Verification items for the finished model (mm, model axes). A direction names the side the tool comes from. Coordinates: 2 decimals unless noted, no trailing zeros. Loops run counter-clockwise (first coordinate to the right, second up) from the corner with the lowest first, then second, coordinate; pieces in that order, holes last. Notation, with made-up numbers: (-31.5, 41) - (-10.5, 41) arc R15 ccw to (-10.5, 52) - close; hole circle Ø5 at (20.25, 62). An arc over 180 degrees is marked (long way). Answer as CSV lines item,"result". Start each with the question number.
1. Cross-section at C-C (z = 45.5). Enter the section's corners in (x, y), plus the area to 3 significant figures.
2. Cross-section at A-A (z = 0). Enter the section's corners in (x, y), plus the area to 3 significant figures.
3. Set-up check for faces 5 (the flat face through (-63.292, -153, 29)), 6 (the flat face through (-54.96, -150.6, 51.33)), 7 (the flat face through (-63.292, -153, -30)), 8 (the flat face through (-65, -150, 0)): record each of +Z, -Z, +X, -X, +Y, -Y from which the full face is reachable in a straight line by a thin tool's end or side.
4. Gauge pin test, flat ends, axial feed: P1, Ø4, axis at x = -101, y = -151, coming from the -Z side; P2, Ø4, axis at x = -56.29, z = 50, coming from the +Y side; P3, Ø1.8, axis at x = -56, z = -9, coming from the -Y side; P4, Ø11, axis at x = -56.29, z = 0, coming from the -Y side. Record the tip position at first contact, or that the pin passes through.
5. Material ranges on line 1 (X direction, y = -149.65, z = 0); line 2 (X direction, y = -153.95, z = 0); line 3 (X direction, y = -150.15, z = 0), recorded low to high. Write a range as [from, to].
6. Release check for a two-part mould opening along Z. For faces 1 (the cylindrical face through (-56.4, -153.1, 57)), 2 (the cylindrical face through (-109.32, -149.81, -0.67)), 3 (the flat face through (-49.292, -153, -29)), 4 (the flat face through (-85, -153, -7)) record: pulls with the +Z half, pulls with the -Z half, needs draft (parallel to the pull), parting line crosses it, or undercut.
7. Cross-section at B-B (x = -72). Enter the section's corners in (y, z).
```python
from build123d import *

# Parameters (mm, degrees)
BASE_OUTLINE_SKETCH_R          = 1.7
BASE_OUTLINE_SKETCH_R_2        = 6.1
BASE_OUTLINE_SKETCH_R_3        = 1.6
BASE_OUTLINE_DEPTH             = 4
INTERFACE_PROFILE_2_SKETCH_R   = 1.7
INTERFACE_PROFILE_2_SKETCH_R_2 = 6.1
INTERFACE_PROFILE_2_SKETCH_R_3 = 1.1
INTERFACE_PROFILE_2_DEPTH      = 2.4
INTERFACE_PROFILE_3_SKETCH_R   = 6.1
INTERFACE_PROFILE_3_SKETCH_R_2 = 3.1
INTERFACE_PROFILE_3_SKETCH_R_3 = 1.1
INTERFACE_PROFILE_3_DEPTH      = 0.6
INTERFACE_PROFILE_4_SKETCH_R   = 6.1
INTERFACE_PROFILE_4_SKETCH_R_2 = 3.1
INTERFACE_PROFILE_4_DEPTH      = 1


with BuildPart() as part:
    # Base Outline Sketch → Base Outline (new body)
    with BuildSketch(Plane(origin=(0, -157, 0), x_dir=(1, 0, 0), z_dir=(0, 1, 0))):
        with BuildLine():
            Line((-106.291651246, -7), (-64.77693262, -7))
            ThreePointArc((-64.77693262, -7), (-64.069825839, -7.778174593), (-63.291651246, -8.485281374))
            Line((-63.291651246, -8.485281374), (-63.291651246, -50))
            ThreePointArc((-63.291651246, -50), (-56.291651246, -57), (-49.291651246, -50))
            Line((-49.291651246, -50), (-49.291651246, -8.485281374))
            ThreePointArc((-49.291651246, -8.485281374), (-45.291651246, 0), (-49.291651246, 8.485281374))
            Line((-49.291651246, 8.485281374), (-49.291651246, 50))
            ThreePointArc((-49.291651246, 50), (-56.291651246, 57), (-63.291651246, 50))
            Line((-63.291651246, 50), (-63.291651246, 8.485281374))
            ThreePointArc((-63.291651246, 8.485281374), (-64.069825839, 7.778174593), (-64.77693262, 7))
            Line((-64.77693262, 7), (-106.291651246, 7))
            ThreePointArc((-106.291651246, 7), (-113.291651246, 0), (-106.291651246, -7))
        make_face()
        with Locations(Location((-106.291651246, 0, 0), (0, 0, 270))):
            Circle(BASE_OUTLINE_SKETCH_R, mode=Mode.SUBTRACT)
        with Locations(Location((-56.291651246, 50, 0), (0, 0, 270))):
            Circle(BASE_OUTLINE_SKETCH_R, mode=Mode.SUBTRACT)
        with Locations(Location((-56.291651246, 0, 0), (0, 0, 270))):
            Circle(BASE_OUTLINE_SKETCH_R_2, mode=Mode.SUBTRACT)
        with Locations(Location((-56.291651246, -50, 0), (0, 0, 270))):
            Circle(BASE_OUTLINE_SKETCH_R, mode=Mode.SUBTRACT)
        with Locations(Location((-65.291651246, 0, 0), (0, 0, 270))):
            Circle(BASE_OUTLINE_SKETCH_R_3, mode=Mode.SUBTRACT)
        with Locations(Location((-56.291651246, -9, 0), (0, 0, 270))):
            Circle(BASE_OUTLINE_SKETCH_R_3, mode=Mode.SUBTRACT)
        with Locations(Location((-56.291651246, 9, 0), (0, 0, 270))):
            Circle(BASE_OUTLINE_SKETCH_R_3, mode=Mode.SUBTRACT)
    extrude(amount=BASE_OUTLINE_DEPTH)

    # Interface Profile 2 Sketch → Interface Profile 2 (add)
    with BuildSketch(Plane(origin=(0, -153, 0), x_dir=(1, 0, 0), z_dir=(0, 1, 0))):
        with BuildLine():
            Line((-106.291651246, -7), (-64.77693262, -7))
            ThreePointArc((-64.77693262, -7), (-64.069825839, -7.778174593), (-63.291651246, -8.485281374))
            Line((-63.291651246, -8.485281374), (-63.291651246, -50))
            ThreePointArc((-63.291651246, -50), (-56.291651246, -57), (-49.291651246, -50))
            Line((-49.291651246, -50), (-49.291651246, -8.485281374))
            ThreePointArc((-49.291651246, -8.485281374), (-45.291651246, 0), (-49.291651246, 8.485281374))
            Line((-49.291651246, 8.485281374), (-49.291651246, 50))
            ThreePointArc((-49.291651246, 50), (-56.291651246, 57), (-63.291651246, 50))
            Line((-63.291651246, 50), (-63.291651246, 8.485281374))
            ThreePointArc((-63.291651246, 8.485281374), (-64.069825839, 7.778174593), (-64.77693262, 7))
            Line((-64.77693262, 7), (-106.291651246, 7))
            ThreePointArc((-106.291651246, 7), (-113.291651246, 0), (-106.291651246, -7))
        make_face()
        with Locations(Location((-106.291651246, 0, 0), (0, 0, 270))):
            Circle(INTERFACE_PROFILE_2_SKETCH_R, mode=Mode.SUBTRACT)
        with Locations(Location((-56.291651246, 50, 0), (0, 0, 270))):
            Circle(INTERFACE_PROFILE_2_SKETCH_R, mode=Mode.SUBTRACT)
        with Locations(Location((-56.291651246, 0, 0), (0, 0, 270))):
            Circle(INTERFACE_PROFILE_2_SKETCH_R_2, mode=Mode.SUBTRACT)
        with Locations(Location((-56.291651246, -50, 0), (0, 0, 270))):
            Circle(INTERFACE_PROFILE_2_SKETCH_R, mode=Mode.SUBTRACT)
        with Locations(Location((-65.291651246, 0, 0), (0, 0, 270))):
            Circle(INTERFACE_PROFILE_2_SKETCH_R_3, mode=Mode.SUBTRACT)
        with Locations(Location((-56.291651246, -9, 0), (0, 0, 270))):
            Circle(INTERFACE_PROFILE_2_SKETCH_R_3, mode=Mode.SUBTRACT)
        with Locations(Location((-56.291651246, 9, 0), (0, 0, 270))):
            Circle(INTERFACE_PROFILE_2_SKETCH_R_3, mode=Mode.SUBTRACT)
    extrude(amount=INTERFACE_PROFILE_2_DEPTH)

    # Interface Profile 3 Sketch → Interface Profile 3 (add)
    with BuildSketch(Plane(origin=(0, -150.6, 0), x_dir=(1, 0, 0), z_dir=(0, 1, 0))):
        with BuildLine():
            Line((-106.291651246, -7), (-64.77693262, -7))
            ThreePointArc((-64.77693262, -7), (-64.069825839, -7.778174593), (-63.291651246, -8.485281374))
            Line((-63.291651246, -8.485281374), (-63.291651246, -50))
            ThreePointArc((-63.291651246, -50), (-56.291651246, -57), (-49.291651246, -50))
            Line((-49.291651246, -50), (-49.291651246, -8.485281374))
            ThreePointArc((-49.291651246, -8.485281374), (-45.291651246, 0), (-49.291651246, 8.485281374))
            Line((-49.291651246, 8.485281374), (-49.291651246, 50))
            ThreePointArc((-49.291651246, 50), (-56.291651246, 57), (-63.291651246, 50))
            Line((-63.291651246, 50), (-63.291651246, 8.485281374))
            ThreePointArc((-63.291651246, 8.485281374), (-64.069825839, 7.778174593), (-64.77693262, 7))
            Line((-64.77693262, 7), (-106.291651246, 7))
            ThreePointArc((-106.291651246, 7), (-113.291651246, 0), (-106.291651246, -7))
        make_face()
        with Locations(Location((-56.291651246, 0, 0), (0, 0, 270))):
            Circle(INTERFACE_PROFILE_3_SKETCH_R, mode=Mode.SUBTRACT)
        with Locations(Location((-106.291651246, 0, 0), (0, 0, 270))):
            Circle(INTERFACE_PROFILE_3_SKETCH_R_2, mode=Mode.SUBTRACT)
        with Locations(Location((-56.291651246, 50, 0), (0, 0, 270))):
            Circle(INTERFACE_PROFILE_3_SKETCH_R_2, mode=Mode.SUBTRACT)
        with Locations(Location((-56.291651246, -50, 0), (0, 0, 270))):
            Circle(INTERFACE_PROFILE_3_SKETCH_R_2, mode=Mode.SUBTRACT)
        with Locations(Location((-65.291651246, 0, 0), (0, 0, 270))):
            Circle(INTERFACE_PROFILE_3_SKETCH_R_3, mode=Mode.SUBTRACT)
        with Locations(Location((-56.291651246, -9, 0), (0, 0, 270))):
            Circle(INTERFACE_PROFILE_3_SKETCH_R_3, mode=Mode.SUBTRACT)
        with Locations(Location((-56.291651246, 9, 0), (0, 0, 270))):
            Circle(INTERFACE_PROFILE_3_SKETCH_R_3, mode=Mode.SUBTRACT)
    extrude(amount=INTERFACE_PROFILE_3_DEPTH)

    # Interface Profile 4 Sketch → Interface Profile 4 (add)
    with BuildSketch(Plane(origin=(0, -150, 0), x_dir=(1, 0, 0), z_dir=(0, 1, 0))):
        with BuildLine():
            Line((-106.291651246, -7), (-64.77693262, -7))
            ThreePointArc((-64.77693262, -7), (-64.069825839, -7.778174593), (-63.291651246, -8.485281374))
            Line((-63.291651246, -8.485281374), (-63.291651246, -50))
            ThreePointArc((-63.291651246, -50), (-56.291651246, -57), (-49.291651246, -50))
            Line((-49.291651246, -50), (-49.291651246, -8.485281374))
            ThreePointArc((-49.291651246, -8.485281374), (-45.291651246, 0), (-49.291651246, 8.485281374))
            Line((-49.291651246, 8.485281374), (-49.291651246, 50))
            ThreePointArc((-49.291651246, 50), (-56.291651246, 57), (-63.291651246, 50))
            Line((-63.291651246, 50), (-63.291651246, 8.485281374))
            ThreePointArc((-63.291651246, 8.485281374), (-64.069825839, 7.778174593), (-64.77693262, 7))
            Line((-64.77693262, 7), (-106.291651246, 7))
            ThreePointArc((-106.291651246, 7), (-113.291651246, 0), (-106.291651246, -7))
        make_face()
        with Locations(Location((-56.291651246, 0, 0), (0, 0, 270))):
            Circle(INTERFACE_PROFILE_4_SKETCH_R, mode=Mode.SUBTRACT)
        with Locations(Location((-106.291651246, 0, 0), (0, 0, 270))):
            Circle(INTERFACE_PROFILE_4_SKETCH_R_2, mode=Mode.SUBTRACT)
        with Locations(Location((-56.291651246, 50, 0), (0, 0, 270))):
            Circle(INTERFACE_PROFILE_4_SKETCH_R_2, mode=Mode.SUBTRACT)
        with Locations(Location((-56.291651246, -50, 0), (0, 0, 270))):
            Circle(INTERFACE_PROFILE_4_SKETCH_R_2, mode=Mode.SUBTRACT)
    extrude(amount=INTERFACE_PROFILE_4_DEPTH)


solid = part.part
```
Values follow:
1,outline,"(-63.29, -157) - (-49.29, -157) - (-49.29, -149) - (-63.29, -149) - close"
1,area,"112 mm²"
2,outline,"(-113.29, -157) - (-107.99, -157) - (-107.99, -150.6) - (-109.39, -150.6) - (-109.39, -149) - (-113.29, -149) - close; (-104.59, -157) - (-66.89, -157) - (-66.89, -153) - (-66.39, -153) - (-66.39, -150) - (-64.19, -150) - (-64.19, -153) - (-63.69, -153) - (-63.69, -157) - (-62.39, -157) - (-62.39, -149) - (-103.19, -149) - (-103.19, -150.6) - (-104.59, -150.6) - close; (-50.19, -157) - (-45.29, -157) - (-45.29, -149) - (-50.19, -149) - close"
2,area,"395 mm²"
3,face 5,"+Z, -X, +Y, -Y"
3,face 6,"+Y"
3,face 7,"-Z, -X, +Y, -Y"
3,face 8,"-Y"
4,P1,"stops at z = -7"
4,P2,"stops at y = -150.6"
4,P3,"stops at y = -153"
4,P4,"passes through"
5,line 1,"x = [-113.29, -109.39], [-103.19, -62.39], [-50.19, -45.29]"
5,line 2,"x = [-113.29, -107.99], [-104.59, -66.89], [-63.69, -62.39], [-50.19, -45.29]"
5,line 3,"x = [-113.29, -109.39], [-103.19, -66.39], [-64.19, -62.39], [-50.19, -45.29]"
6,face 1,"pulls with the +Z half"
6,face 2,"undercut"
6,face 3,"needs draft"
6,face 4,"pulls with the -Z half"
7,outline,"(-157, -7) - (-149, -7) - (-149, 7) - (-157, 7) - close"
